```python
from build123d import *

# Parameters (mm, degrees)
EURO_CYLINDER_OUTLINE_DEPTH = 44.5
SKETCH9_R                   = 7.25
BORE_FOR_CORE_DEPTH         = 37
SKETCH2_R                   = 1
HOLE_FOR_PIN_DEPTH          = 35
LPATTERN_OF_6_COUNT         = 6
LPATTERN_OF_6_PITCH         = 4.25
OPENNING_DEPTH              = 53.422705051
OPENNING_DEPTH_BACK         = 53.422705051
SKETCH3_W                   = 9.25
SKETCH3_H                   = 24
F_0_5_X_45_DEG_SIZE         = 0.5
SKETCH10_R                  = 6.5
DIA_13_END_BIT_DEPTH        = 49.786678644


with BuildPart() as part:
    # Sketch1 → euro cylinder outline (new body)
    with BuildSketch(Plane(origin=(0, 0, 0), x_dir=(0, 0, -1), z_dir=(1, 0, 0))):
        with BuildLine():
            Line((-5, 19.5), (-5, 6.873863542))
            ThreePointArc((-5, 6.873863542), (0, -8.5), (5, 6.873863542))
            Line((5, 6.873863542), (5, 19.5))
            ThreePointArc((5, 19.5), (4.094469505, 22.369724634), (1.705872211, 24.2))
            Line((1.705872211, 24.2), (-1.705872211, 24.2))
            ThreePointArc((-1.705872211, 24.2), (-4.094469505, 22.369724634), (-5, 19.5))
        make_face()
    extrude(amount=EURO_CYLINDER_OUTLINE_DEPTH)

    # Sketch9 → bore for core (cut)
    with BuildSketch(Plane.ZY):
        Circle(SKETCH9_R)
    extrude(amount=-BORE_FOR_CORE_DEPTH, mode=Mode.SUBTRACT)

    # Sketch2 → hole for pin (cut)
    with BuildSketch(Plane(origin=(0, 0, 0), x_dir=(1, 0, 0), z_dir=(0, 1, 0))):
        with Locations(Location((5, 0, 0), (0, 0, 90))):
            Circle(SKETCH2_R)
    hole_for_pin = extrude(amount=HOLE_FOR_PIN_DEPTH, mode=Mode.SUBTRACT)

    # LPattern of 6: hole for pin ×6
    with Locations(*[(i * LPATTERN_OF_6_PITCH, 0, 0) for i in range(1, LPATTERN_OF_6_COUNT)]):
        add(hole_for_pin, mode=Mode.SUBTRACT)

    # Sketch3 → openning (cut, two sides: drawn at the far end of the back side and taken through both)
    with BuildSketch(Plane.XY.offset(5).offset(-OPENNING_DEPTH_BACK)):
        with Locations((36.875, 3.5)):
            Rectangle(SKETCH3_W, SKETCH3_H)
    extrude(amount=OPENNING_DEPTH + OPENNING_DEPTH_BACK, mode=Mode.SUBTRACT)

    # Sketch7 → M5x0.8 mounting hole (revolve, cut)
    with BuildSketch(Plane(origin=(37, 19.5, 5), x_dir=(0, -1, 0), z_dir=(1, 0, 0))):
        Polygon((0, 0), (0, 10), (3, 10), (2.1, 9.1), (2.1, 0.9), (3, 0), align=None)
    revolve(axis=Axis((37, 19.5, 11.35), (0, 0, -1)), mode=Mode.SUBTRACT)

    # 0.5 x 45 deg
    f_0_5_x_45_deg_edges = [part.edges().sort_by_distance(p)[0] for p in [
        (0, 24.2, 0),
    ]]
    chamfer(f_0_5_x_45_deg_edges, length=F_0_5_X_45_DEG_SIZE)
    f_0_5_x_45_deg_2_edges = [part.edges().sort_by_distance(p)[0] for p in [
        (0, 21.891164992, -4.391164992),
        (0, 13.186931771, -5),
    ]]
    chamfer(f_0_5_x_45_deg_2_edges, length=F_0_5_X_45_DEG_SIZE)
    f_0_5_x_45_deg_3_edges = [part.edges().sort_by_distance(p)[0] for p in [
        (0, 21.891164992, 4.391164992),
        (0, 13.186931771, 5),
    ]]
    chamfer(f_0_5_x_45_deg_3_edges, length=F_0_5_X_45_DEG_SIZE)
    f_0_5_x_45_deg_4_edges = [part.edges().sort_by_distance(p)[0] for p in [
        (0, -8.5, 0),
    ]]
    chamfer(f_0_5_x_45_deg_4_edges, length=F_0_5_X_45_DEG_SIZE - 0.0001)  # a hair under: the kernel refuses the full size

    # Sketch10 → dia 13 end bit (cut, through all)
    with BuildSketch(Plane.ZY.offset(-41.5)):
        Circle(SKETCH10_R)
    extrude(amount=-DIA_13_END_BIT_DEPTH, mode=Mode.SUBTRACT)


solid = part.part
```
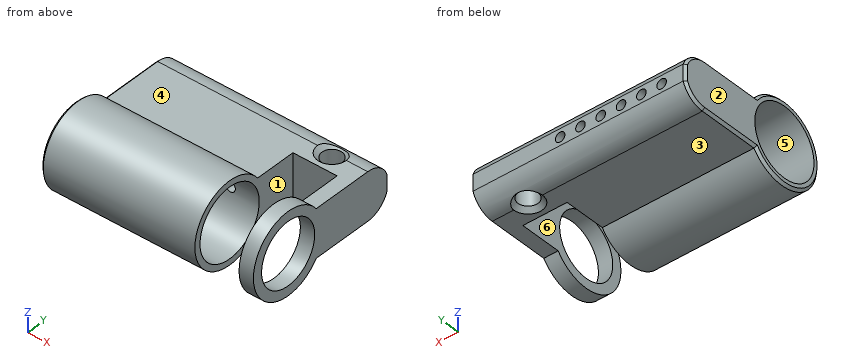
Build history of the part. All positions in model axes, mm. Face numbers are marked on the shaded views. A direction names the side the tool comes from. Coordinates: 2 decimals unless noted, no trailing zeros. Order: outer loops, then holes, each group sorted by start corner. A loop starts at its lowest first (then second) coordinate and runs counter-clockwise, first axis right, second up.
Item 1: Saw through at A-A on x = 16. List the corners of the cut face in (y, z), then the cut area to 3 significant figures.
Filled in:
outline: (6.87, -5) - (19.5, -5) arc R5 ccw to (24.2, -1.71) - (24.2, 1.71) arc R5 ccw to (19.5, 5) - (6.87, 5) arc R8.5 ccw (long way) to start; hole circle Ø14.5 at (0, 0)
area: 216 mm2
Item 2: Saw through at D-D on x = 37. List the corners of the cut face in (y, z).
Filled in:
outline: (15.5, -5) - (16.5, -5) - (17.4, -4.1) - (17.4, 4.1) - (16.5, 5) - (15.5, 5) - close; (21.6, -4.1) - (21.89, -4.39) arc R5 ccw to (24.2, -1.71) - (24.2, 1.71) arc R5 ccw to (21.89, 4.39) - (21.6, 4.1) - close
Item 3: Mould opens along Z. For the marked faces 4, 5 and 6 say: released by +Z, released by -Z, zero draft, split by the parting line, or undercut.
Filled in:
face 4: released by +Z
face 5: undercut
face 6: zero draft
Item 4: Drop flat-ended pins along their axis: pin 1 Ø5 at (y, z) = (-2, -4) entering from -X; pin 2 Ø6.5 at (x, y) = (16.5, 16) entering from +Z; pin 3 Ø12 at (x, y) = (29.5, 12) entering from -Z. Give the stop position or say it passes through.
Filled in:
pin 1: stops at x = 41.5
pin 2: stops at z = 5
pin 3: stops at z = -6.02
Item 5: Drill centre lines: L1, parallel to Z at x = 13.5, y = 14.75; L2, parallel to X at y = 4.5, z = 6.25; L3, parallel to X at y = 19.5, z = 1.75. Where is each one in solid material? Low to high.
Filled in:
L1: z = -5 to -1, 1 to 5
L2: x = 0 to 32.25, 41.5 to 44.5
L3: x = 0 to 34.9, 39.1 to 44.5
Item 6: Saw through at B-B on x = 26.25. List the corners of the cut face in (y, z).
Filled in:
outline: (6.87, -5) - (19.5, -5) arc R5 ccw to (24.2, -1.71) - (24.2, -1) - (7.18, -1) arc R7.25 cw (long way) to (7.18, 1) - (24.2, 1) - (24.2, 1.71) arc R5 ccw to (19.5, 5) - (6.87, 5) arc R8.5 ccw (long way) to start
Item 7: Saw through at C-C on z = 0. State how many separate pieces and enclosed holes the cut face has, then the cut area to 3 significant figures.
Filled in:
separate pieces: 9
enclosed holes: 1
area: 509 mm2
Item 8: Tool access for the marked faces 1, 2 and 3: list every direction of +Z, -Z, +X, -X, +Y, -Y with a clear straight run to the whole face (end or side of a thin tool).
Filled in:
face 1: +Z, -Z, -Y
face 2: +Z, -Z, -X, +Y, -Y
face 3: -Z, +X, -X, +Y
